Check sheet for the modelled part. Datum: model origin and axes. Units: mm. Coordinates: 2 decimals unless noted, no trailing zeros. Loops run counter-clockwise (first coordinate to the right, second up) from the corner with the lowest first, then second, coordinate; pieces in that order, holes last. Notation, with made-up numbers: M 46.25,48.5 L 85.25,48.5 A23 ccw 85.25,76.5 Z; hole C -28.75,60.25 d7. An arc over 180 degrees is marked long. Return JSON: item names as keys, results as strings.
from build123d import *

# Parameters (mm, degrees)
SKETCH_W   = 185
SKETCH_H   = 86
SKETCH_R   = 11.8
SKETCH_R_2 = 1.55
SKETCH_R_3 = 1.6
SKETCH_W_2 = 9.78
SKETCH_H_2 = 27.68
PAD_DEPTH  = 3


with BuildPart() as part:
    # Sketch → Pad (new body)
    with BuildSketch(Plane.YZ):
        Rectangle(SKETCH_W, SKETCH_H)
        with Locations((68.2497, -5)):
            Circle(SKETCH_R, mode=Mode.SUBTRACT)
        with Locations((80.2497, 4.5)):
            Circle(SKETCH_R_2, mode=Mode.SUBTRACT)
        with Locations((56.2497, -14.5)):
            Circle(SKETCH_R_2, mode=Mode.SUBTRACT)
        with Locations((21.6847, 5.795)):
            Circle(SKETCH_R_3, mode=Mode.SUBTRACT)
        with Locations((21.6847, -15.795)):
            Circle(SKETCH_R_3, mode=Mode.SUBTRACT)
        with Locations((-50.7053, 5.795)):
            Circle(SKETCH_R_3, mode=Mode.SUBTRACT)
        with Locations((-50.7053, -15.795)):
            Circle(SKETCH_R_3, mode=Mode.SUBTRACT)
        with Locations((12.7947, -5)):
            Rectangle(SKETCH_W_2, SKETCH_H_2, mode=Mode.SUBTRACT)
    extrude(amount=PAD_DEPTH)


solid = part.part
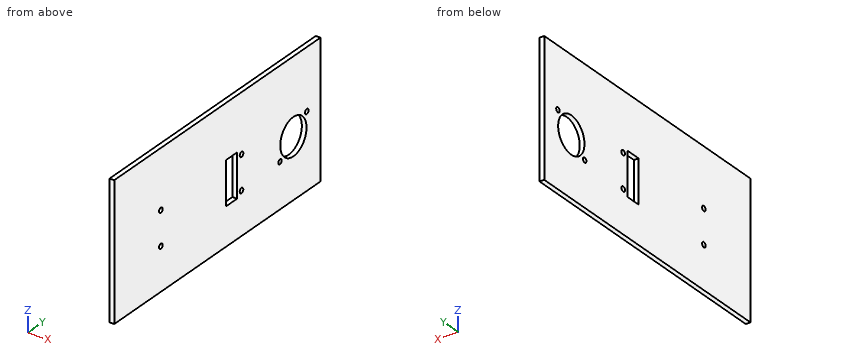
1) Section check B-B on y = 13.5. Record the cut outline in (x, z).
Answers:
{"outline": "M 0,-43 L 3,-43 L 3,-18.84 L 0,-18.84 Z; M 0,8.84 L 3,8.84 L 3,43 L 0,43 Z"}
2) Scan lines: line 1 along Z through (x, y) = (1.5, -51); line 2 along Z through (x, y) = (1.15, 16); line 3 along Y through (x, z) = (2.5, -9.5). Record each from-to range of solid material in increasing order. Write a range as [from, to].
Answers:
{"line 1": "[-43, -17.37], [-14.22, 4.22], [7.37, 43]", "line 2": "[-43, -18.84], [8.84, 43]", "line 3": "[-92.5, 7.9], [17.68, 57.34], [79.16, 92.5]"}
3) Section check A-A on z = -5. Record the cut outline in (x, y), then the cut area to 3 significant figures.
Answers:
{"outline": "M 0,-92.5 L 3,-92.5 L 3,7.9 L 0,7.9 Z; M 0,17.68 L 3,17.68 L 3,56.45 L 0,56.45 Z; M 0,80.05 L 3,80.05 L 3,92.5 L 0,92.5 Z", "area": "455 mm²"}
4) Section check C-C on x = 2.3. Count the separate pieces of the cut face and the enclosed holes in it, then the cut area to 3 significant figures.
Answers:
{"separate pieces": "1", "enclosed holes": "8", "area": "15,200 mm²"}
